The model under review builds one solid part; all positions refer to its coordinate system, in mm. Give positions to 0.01 mm unless a question says otherwise; leave off trailing zeros. Order: outer loops, then holes, each group sorted by start corner. A loop starts at its lowest first (then second) coordinate and runs counter-clockwise, first axis right, second up. Notation, with made-up numbers: M -28,42.5 L -5,42.5 A21 cw -5,51.5 Z; hole C 84.5,68.25 d2. An arc over 180 degrees is marked long. One line per question, with ' | ' between items. Start each with the question number.
1. We need section C-C on z = 85. Write out the cut boundary in (x, y), then the cut area to 3 significant figures.
2. We need section A-A on x = 77. Write out the cut boundary in (y, z).
3. We need section B-B on y = 3.35. Write out the cut boundary in (x, z), then the cut area to 3 significant figures.
4. Insertion check: P1, Ø1.5, axis at x = -135.5, z = -201.5, coming from the -Y side; P2, Ø2, axis at y = 1.5, z = -32.5, coming from the -X side. Each pin has a flat end and moves straight along its axis. Give the tip position at first contact, or say it passes through.
5. Wall thickness on L1, parallel to Z at x = 98, y = 1.7; L2, parallel to X at y = 2.8, z = -96.5; L3, parallel to X at y = 2.95, z = 12: over which ranges is each line inside the solid? List them lowest first.
```python
from build123d import *

# Parameters (mm, degrees)
SKETCH_1_W          = 400
SKETCH_1_H          = 600
EXTRUDE_1_DEPTH     = 4
SKETCH_2_W          = 140
SKETCH_2_H          = 210
CUT_EXTRUDE_3_DEPTH = 361.577314872
FILLET_1_R          = 10


with BuildPart() as part:
    # 草图1 → 凸台-拉伸1 (new body)
    with BuildSketch(Plane(origin=(0, 0, 0), x_dir=(1, 0, 0), z_dir=(0, 1, 0))):
        Rectangle(SKETCH_1_W, SKETCH_1_H)
    extrude(amount=EXTRUDE_1_DEPTH)

    # 草图2 → 切除-拉伸3 (cut, through all)
    with BuildSketch(Plane(origin=(0, 4, 0), x_dir=(1, 0, 0), z_dir=(0, 1, 0))):
        with Locations((-130, 0)):
            Rectangle(SKETCH_2_W, SKETCH_2_H)
    cut_extrude_3 = extrude(amount=-CUT_EXTRUDE_3_DEPTH, mode=Mode.SUBTRACT)

    # 镜向1: 切除-拉伸3 across plane
    add(cut_extrude_3.mirror(Plane(origin=(0, 0, 0), x_dir=(0, 0, 1), z_dir=(1, 0, 0))), mode=Mode.SUBTRACT)

    # 圆角1
    fillet_1_edges = [part.edges().sort_by_distance(p)[0] for p in [
        (-60, 2, -105),
        (-60, 2, 105),
        (-200, 2, 105),
        (-200, 2, -105),
        (60, 2, 105),
        (60, 2, -105),
        (200, 2, -105),
        (200, 2, 105),
    ]]
    fillet(fillet_1_edges, radius=FILLET_1_R)


solid = part.part
```
Entries:
1) outline: M -60,0 L 60,0 L 60,4 L -60,4 Z | area: 480 mm^2
2) outline: M 0,-300 L 4,-300 L 4,-105 L 0,-105 Z; M 0,105 L 4,105 L 4,300 L 0,300 Z
3) outline: M -200,-300 L 200,-300 L 200,-115 A10 ccw 190,-105 L 70,-105 A10 cw 60,-95 L 60,95 A10 cw 70,105 L 190,105 A10 ccw 200,115 L 200,300 L -200,300 L -200,115 A10 ccw -190,105 L -70,105 A10 cw -60,95 L -60,-95 A10 cw -70,-105 L -190,-105 A10 ccw -200,-115 Z | area: 181,000 mm^2
4) P1: stops at y = 0 | P2: stops at x = -60
5) L1: z = -300 to -105, 105 to 300 | L2: x = -60.11 to 60.11 | L3: x = -60 to 60
